Part model, mm, in its own coordinate system. Give positions to 0.01 mm unless a question says otherwise; leave off trailing zeros. Write each loop counter-clockwise with the first axis right and the second up, starting at its lowest first coordinate (ties: lowest second). Pieces come first, ordered by that corner, then holes. Notation, with made-up numbers: (44.25, 37) - (102.25, 37) arc R19 ccw to (102.25, 60) - close; hole circle Ø2 at (42, 55). An arc over 180 degrees is marked (long way). Answer in a Markdown table with one row per item. Add a question column.
1. Band-saw the part on B-B on y = 125. Write the cut outline in (x, z).
2. Band-saw the part on A-A on x = 75. Write the cut outline in (y, z).
3. Probe line 1 along Y through (x, z) = (75, 31); line 2 along X through (y, z) = (125, 15); line 3 along X through (y, z) = (130, 15.5). List the from-to ranges inside material, lowest first.
4. Pull direction Y, two halves, no side cores. Call faces 1 (the flat face through (740, 0, 25)), 2 (the conical face through (65.682, 137.152, 45.313)), 3 (the conical face through (1409.82, 126.99, 4.69)), 4 (the flat face through (740, 101, 50)): released by +Y, released by -Y, zero draft, split by the parting line, or undercut.
5. Drop a flat-ended pin along its axis: pin 1 Ø2 at (y, z) = (145, 42.5) entering from -X. Give the stop position or say it passes through.
Autodesk Inventor part; units mm, degrees
ref_plane "YZ Plane" through (0, 0, 0) normal (1, 0, 0) x (0, 1, 0)
ref_plane "XZ Plane" through (0, 0, 0) normal (0, 1, 0) x (-1, 0, 0)
ref_plane "XY Plane" through (0, 0, 0) normal (0, 0, 1) x (1, 0, 0)
sketch "Sketch1" plane through (0, 0, 0) normal (0, 0, 1) x (1, 0, 0)
  line L0 (0, 0) -> (1500, 0)
  line L1 (1500, 0) -> (1500, 200)
  line L2 (1500, 200) -> (0, 200)
  line L3 (0, 200) -> (0, 0)
  dimension "d0" = 200
  dimension "d1" = 1500
extrude "Extrusion1" add sketch "Sketch1" along normal blind 50
sketch "Sketch2" plane through (0, 0, 50) normal (0, 0, 1) x (1, 0, 0)
  line L0 (0, 200) -> (0, 0)
  line L1 (1500, 0) -> (1500, 200)
  line L2 (1500, 200) -> (0, 200)
  point P0 (75, 125)
  point P1 (1425, 125)
  point P2 (0, 100)
  dimension "d4" = 75
  dimension "d5" = 75
  dimension "d19" = 75
hole "Hole1" at (75, 125, 50) at (1425, 125, 50) direction (0, 0, -1) diameter 30 end through all
chamfer "Chamfer1" distance 5 angle 45 4 edges at (75, 140, 50) (1425, 140, 50) (75, 140, 0) (1425, 140, 0)
chamfer "Chamfer2" distance 100 angle 30 1 edges at (1500, 200, 25) measured on face at (1500, 66.6667, 16.6667)
properties part number "Top_Floor Plank" material "Wood (Birch)"
Values:
| question | item | result |
|---|---|---|
| 1 | outline | (0, 0) - (55, 0) - (60, 5) - (60, 45) - (55, 50) - (0, 50) - close; (90, 5) - (95, 0) - (1405, 0) - (1410, 5) - (1410, 45) - (1405, 50) - (95, 50) - (90, 45) - close; (1440, 5) - (1445, 0) - (1485.57, 0) - (1485.57, 50) - (1445, 50) - (1440, 45) - close |
| 2 | outline | (0, 0) - (105, 0) - (110, 5) - (110, 45) - (105, 50) - (0, 50) - close; (140, 5) - (145, 0) - (200, 0) - (200, 50) - (145, 50) - (140, 45) - close |
| 3 | line 1 | y = 0 to 110, 140 to 200 |
| 3 | line 2 | x = 0 to 60, 90 to 1410, 1440 to 1485.57 |
| 3 | line 3 | x = 0 to 60.86, 89.14 to 1410.86, 1439.14 to 1482.68 |
| 4 | face 1 | released by -Y |
| 4 | face 2 | undercut |
| 4 | face 3 | undercut |
| 4 | face 4 | zero draft |
| 5 | pin 1 | stops at x = 0 |
